Read the model definition and answer for the solid it produces. Units are mm, in the model's axes. Face numbers are marked on the shaded views. A direction names the side the tool comes from. Coordinates: 2 decimals unless noted, no trailing zeros. Write each loop counter-clockwise with the first axis right and the second up, starting at its lowest first coordinate (ties: lowest second). Pieces come first, ordered by that corner, then holes.
1) The part is cut by section D-D (z = -13). Determine the outline of the cut face in (x, y).
2) Which of the six approach directions +Z, -Z, +X, -X, +Y, -Y give full straight-line access (tool end or side, diameter ignored) to the marked faces 5, 6, 7, 8 and 9?
3) Determine the mould class of the marked faces 1, 2, 3 and 4 for opening direction X: +X half, -X half, draft (parallel to the pull), parting line (faces both ways), or undercut.
4) Each of these flat-tipped pins is pushed along its axis until it touches: pin 1 Ø3 at (x, y) = (-20, -4) entering from +Z; pin 2 Ø3 at (x, y) = (-20, -25.5) entering from -Z; pin 3 Ø6 at (x, y) = (-17.68, -24.25) entering from +Z (3 decimals); pin 4 Ø4 at (x, y) = (-17.68, 24.25) entering from -Z. Where does it stop, or does it pass through?
5) The part is cut by section B-B (x = 0). Determine the outline of the cut face in (y, z), then the cut area to 3 significant figures.
6) The part is cut by section C-C (y = 16). Determine the outline of the cut face in (x, z).
7) Find the intervals of material crossed by line 1 (Y direction, x = -18.5, z = 12); line 2 (X direction, y = -8, z = 9); line 3 (X direction, y = -26.5, z = -12), in increasing order.
8) The part is cut by section A-A (z = -8). Determine the outline of the cut face in (x, y).
from build123d import *

# Parameters (mm, degrees)
F1_DEPTH       = 35
F3_D           = 5
F3_START       = 1.7550021
F3_CBORE_D     = 10
F3_CBORE_DEPTH = 8
F4_W           = 22.4
F4_H           = 2
F5_DEPTH       = 25


with BuildPart() as f1:
    # F0 (on Front) → F1 (new body, symmetric)
    with BuildSketch(Plane.XZ):
        with BuildLine():
            ThreePointArc((-14.8763772272, 3.3549814595), (15.25, 0), (-14.8763772272, -3.3549814595))
            Line((-14.8763772272, -3.3549814595), (-25.6763772272, -3.3549814595))
            Line((-25.6763772272, -3.3549814595), (-25.6763772272, -11.7549814595))
            ThreePointArc((-25.6763772272, -11.7549814595), (-23.3332314767, -17.411835709), (-17.6763772272, -19.7549814595))
            Line((-17.6763772272, -19.7549814595), (-5.4763772272, -19.7549814595))
            ThreePointArc((-5.4763772272, -19.7549814595), (20.5, 0), (-5.4763772272, 19.7549814595))
            Line((-5.4763772272, 19.7549814595), (-17.6763772272, 19.7549814595))
            ThreePointArc((-17.6763772272, 19.7549814595), (-23.3332314767, 17.411835709), (-25.6763772272, 11.7549814595))
            Line((-25.6763772272, 11.7549814595), (-25.6763772272, 3.3549814595))
            Line((-25.6763772272, 3.3549814595), (-14.8763772272, 3.3549814595))
        make_face()
    extrude(amount=F1_DEPTH, both=True)

    # F3 (through all)
    # its depths count from where the whole tool has entered the part; down to there all is cleared
    with Locations(Plane(origin=(0, 0, -19.7549814595), x_dir=(1, 0, 0), z_dir=(0, 0, -1)).offset(-F3_START)):
        with Locations((-17.6763772272, 24.25), (-17.6763772272, 9.25), (-17.6763772272, -9.25), (-17.6763772272, -24.25)):
            CounterBoreHole(F3_D / 2, F3_CBORE_D / 2, F3_CBORE_DEPTH)

    # F4 (on Top) → F5 (cut, symmetric)
    with BuildSketch(Plane.XY):
        with Locations((-14.4763772272, 0)):
            Rectangle(F4_W, F4_H)
    extrude(amount=F5_DEPTH, both=True, mode=Mode.SUBTRACT)


solid = f1.part
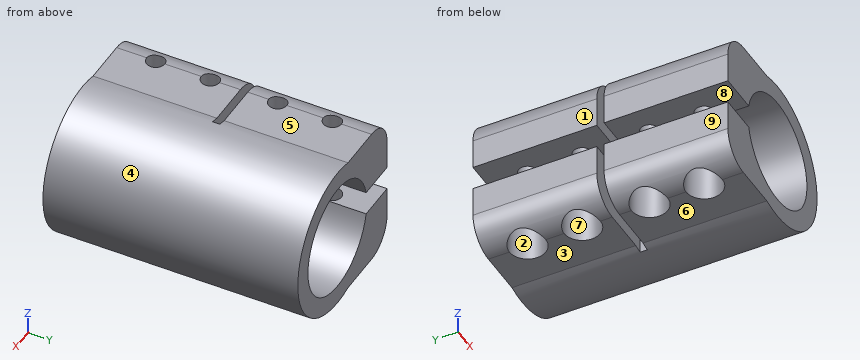
Reported:
1. outline: (-25.58, -35) - (-7.97, -35) - (-7.97, -1) - (-25.58, -1) - close; (-25.58, 1) - (-7.97, 1) - (-7.97, 35) - (-25.58, 35) - close; (7.97, -35) - (15.85, -35) - (15.85, 35) - (7.97, 35) - close; hole circle Ø10 at (-17.68, -24.25); hole circle Ø10 at (-17.68, -9.25); hole circle Ø10 at (-17.68, 9.25); hole circle Ø10 at (-17.68, 24.25)
2. face 5: +Z, -X, +Y, -Y
2. face 6: -Z, -X, +Y, -Y
2. face 7: -Z
2. face 8: -X, +Y, -Y
2. face 9: +Z, -Z, -X, +Y, -Y
3. face 1: -X half
3. face 2: undercut
3. face 3: draft
3. face 4: parting line
4. pin 1: stops at z = 19.71
4. pin 2: stops at z = -10
4. pin 3: stops at z = 19.755
4. pin 4: passes through
5. outline: (-35, -20.5) - (35, -20.5) - (35, -15.25) - (-35, -15.25) - close; (-35, 15.25) - (35, 15.25) - (35, 20.5) - (-35, 20.5) - close
5. area: 735 mm2
6. outline: (-25.68, -11.75) arc R8 ccw to (-17.68, -19.75) - (-5.48, -19.75) arc R20.5 ccw (long way) to (-5.48, 19.75) - (-17.68, 19.75) arc R8 ccw to (-25.68, 11.75) - (-25.68, 3.35) - (-14.88, 3.35) arc R15.25 cw (long way) to (-14.88, -3.35) - (-25.68, -3.35) - close
7. line 1: y = -35 to -26.61, -21.89 to -11.61, -6.89 to -1, 1 to 6.89, 11.61 to 21.89, 26.61 to 35
7. line 2: x = -25.68 to -19.84, -15.51 to -12.31, 12.31 to 18.42
7. line 3: x = -25.67 to -22.14, -13.21 to -9.41, 9.41 to 16.62
8. outline: (-25.68, -35) - (-12.98, -35) - (-12.98, -1) - (-25.68, -1) - close; (-25.68, 1) - (-12.98, 1) - (-12.98, 35) - (-25.68, 35) - close; (12.98, -35) - (18.87, -35) - (18.87, 35) - (12.98, 35) - close; hole circle Ø5 at (-17.68, -24.25); hole circle Ø5 at (-17.68, -9.25); hole circle Ø5 at (-17.68, 9.25); hole circle Ø5 at (-17.68, 24.25)
